```python
from build123d import *

# Parameters (mm, degrees)
F0_W     = 66.970591
F0_H     = 49.764709
F1_DEPTH = 25
F2_R     = 5.663986
F3_R     = 5


with BuildPart() as f1:
    # F0 (on Front) → F1 (new body)
    with BuildSketch(Plane.XZ):
        with Locations((1.852942, 0.926471)):
            Rectangle(F0_W, F0_H)
    extrude(amount=F1_DEPTH)

    # F2
    f2_edges = [f1.edges().sort_by_distance(p)[0] for p in [
        (1.852943, -25, 25.808826),
        (-31.632353, -25, 0.926471),
        (1.852943, -25, -23.955883),
        (35.338238, -25, 0.926471),
    ]]
    fillet(f2_edges, radius=F2_R)

    # F3
    f3_edges = [f1.edges().sort_by_distance(p)[0] for p in [
        (1.852943, 0, 25.808826),
        (-31.632353, 0, 0.926471),
        (1.852943, 0, -23.955883),
        (35.338238, 0, 0.926471),
    ]]
    fillet(f3_edges, radius=F3_R)


solid = f1.part
```
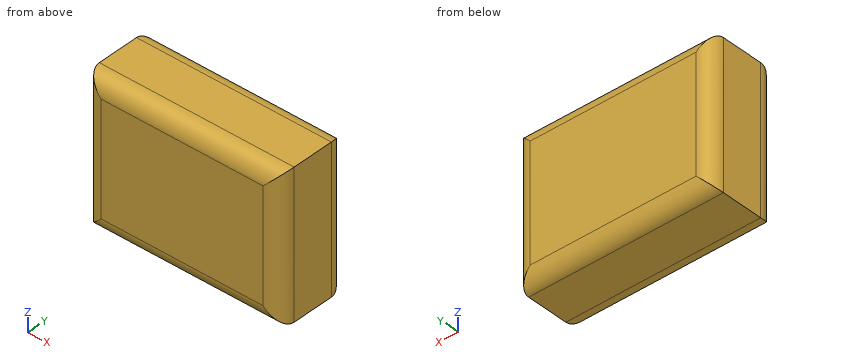
Design review of the part built by this model. Coordinates are the model's own, in mm. Give positions to 0.01 mm unless a question says otherwise; leave off trailing zeros. Loops run counter-clockwise (first coordinate to the right, second up) from the corner with the lowest first, then second, coordinate; pieces in that order, holes last. Notation, with made-up numbers: M -7.75,-2.75 L 51.25,-2.75 A27 cw 51.25,19.25 Z; hole C 82,8.5 d4. An arc over 180 degrees is marked long. Return JSON: item names as keys, results as strings. Group by question number.
Item 1: For probe 1 along Z at (x, y) = (26.5, -2.75); probe 2 along X at (y, z) = (-1.25, -0.5); probe 3 along X at (y, z) = (-21, 8), list the stretches that pass through material, from the lowest coordinate up.
Item 2: We need section A-A (x = 17). Give the boundary of the cut face in (y, z), and give its area (3 significant figures).
Item 3: We need section B-B (y = -3.25). Give the boundary of the cut face in (x, z).
Output:
{
 "1": {"probe 1": "z = -23.42 to 25.27", "probe 2": "x = -29.94 to 33.65", "probe 3": "x = -31.38 to 35.09"},
 "2": {"outline": "M -25,-18.29 A5.66 ccw -19.34,-23.96 L -5,-23.96 A5 ccw 0,-18.96 L 0,20.81 A5 ccw -5,25.81 L -19.34,25.81 A5.66 ccw -25,20.14 Z", "area": "1,220 mm^2"},
 "3": {"outline": "M -31.32,-23.64 L 35.02,-23.64 L 35.02,25.49 L -31.32,25.49 Z"}
}
